```python
from build123d import *

# Parameters (mm, degrees)
F0_W     = 317.5
F0_H     = 57.15
F1_DEPTH = 190.5
F2_W     = 63.5
F2_H     = 31.75
F3_DEPTH = 190.501
F4_W     = 63.5
F4_H     = 31.75
F5_DEPTH = 101.6
F6_W     = 63.5
F6_H     = 127
F7_DEPTH = 127
F9_DEPTH = 57.15


with BuildPart() as f1:
    # F0 (on Front) → F1 (new body)
    with BuildSketch(Plane.XZ):
        with Locations((0, 28.575)):
            Rectangle(F0_W, F0_H)
    extrude(amount=-F1_DEPTH)

    # F2 (on face) → F3 (cut, through all)
    with BuildSketch(Plane.XZ):
        with Locations((-31.75, 15.875)):
            Rectangle(F2_W, F2_H)
    extrude(amount=-F3_DEPTH, mode=Mode.SUBTRACT)

    # F4 (on face) → F5 (cut)
    with BuildSketch(Plane.XZ):
        with Locations((127, 15.875)):
            Rectangle(F4_W, F4_H)
    extrude(amount=-F5_DEPTH, mode=Mode.SUBTRACT)

    # F6 (on face) → F7 (join)
    with BuildSketch(Plane.XY.offset(57.15)):
        with Locations((-127, 127)):
            Rectangle(F6_W, F6_H)
    extrude(amount=F7_DEPTH)

    # F8 (on face) → F9 (join)
    with BuildSketch(Plane.XY.offset(57.15)):
        Polygon((95.25, 190.5), (-95.25, 190.5), (-95.25, 97.55057), (-31.75, 97.55057), (-31.75, 165.1), (31.75, 165.1), (31.75, 97.55057), (95.25, 165.1), align=None)
    extrude(amount=F9_DEPTH)


solid = f1.part
```
Design review of the part built by this model. Coordinates are the model's own, in mm. A direction names the side the tool comes from. Round coordinates to 2 decimals unless told otherwise and drop trailing zeros. Write each loop counter-clockwise with the first axis right and the second up, starting at its lowest first coordinate (ties: lowest second). Pieces come first, ordered by that corner, then holes.
Item 1: The part is to be moulded in two halves that separate along X. For faces 5 (the flat face through (95.25, 50, 16)), 6 (the flat face through (-63.5, 94, 16)), 7 (the flat face through (-112, 94, 0)), say which applies: +X half, -X half, draft (parallel to the pull), parting line (faces both ways), or undercut.
Item 2: We need section D-D on z = 86.5. Write out the cut boundary in (x, y), and give its area (3 significant figures).
Item 3: For probe 1 along X at (y, z) = (110, 14); probe 2 along Z at (x, y) = (-78, 157.5); probe 3 along Z at (x, y) = (63, 50), list the stretches that pass through material, from the lowest coordinate up.
Item 4: Clearance check with flat-ended pins moving along their axes: pin 1 Ø2 at (x, y) = (99.5, 89) entering from +Z; pin 2 Ø6 at (y, z) = (59.5, 23) entering from +X; pin 3 Ø4 at (x, z) = (-45, 42.5) entering from -Y; pin 4 Ø2 at (y, z) = (105.5, 98.5) entering from +X. State where each tip first meets the part, or that it passes through.
Item 5: We need section C-C on x = -25. Write out the cut boundary in (y, z).
Item 6: We need section B-B on y = 86.5. Write out the cut boundary in (x, z).
Item 7: For faces 1 (the flat face through (-31.75, 131, 85)), 2 (the flat face through (127, 101.6, 16)), 3 (the flat face through (63.1, 130.9, 85.3)), 4 (the flat face through (-32, 94, 31.75)), list the 3-axis set-ups (+Z, -Z, +X, -X, +Y, -Y) from which the entire face can be reached by the end or side of a thin tool; tool diameter is ignored.
Item 8: We need section A-A on z = 19. Write out the cut boundary in (x, y).
Returned:
1. face 5: +X half
1. face 6: undercut
1. face 7: draft
2. outline: (-158.75, 63.5) - (-95.25, 63.5) - (-95.25, 97.55) - (-31.75, 97.55) - (-31.75, 165.1) - (31.75, 165.1) - (31.75, 97.55) - (95.25, 165.1) - (95.25, 190.5) - (-158.75, 190.5) - close
2. area: 19,300 mm2
3. probe 1: x = -158.75 to -63.5, 0 to 158.75
3. probe 2: z = 0 to 114.3
3. probe 3: z = 0 to 57.15
4. pin 1: stops at z = 57.15
4. pin 2: stops at x = 95.25
4. pin 3: stops at y = 0
4. pin 4: stops at x = 40.16
5. outline: (0, 31.75) - (190.5, 31.75) - (190.5, 114.3) - (165.1, 114.3) - (165.1, 57.15) - (0, 57.15) - close
6. outline: (-158.75, 0) - (-63.5, 0) - (-63.5, 31.75) - (0, 31.75) - (0, 0) - (95.25, 0) - (95.25, 31.75) - (158.75, 31.75) - (158.75, 57.15) - (-95.25, 57.15) - (-95.25, 184.15) - (-158.75, 184.15) - close
7. face 1: +Z, -Y
7. face 2: -Z, +X, -Y
7. face 3: +Z, +X, -Y
7. face 4: -Z, +Y, -Y
8. outline: (-158.75, 0) - (-63.5, 0) - (-63.5, 190.5) - (-158.75, 190.5) - close; (0, 0) - (95.25, 0) - (95.25, 101.6) - (158.75, 101.6) - (158.75, 190.5) - (0, 190.5) - close
